```python
from build123d import *

# Parameters (mm, degrees)
EXTRU_MINCE1_DEPTH      = 25
CONG_1_R                = 1
CONG_2_R                = 1
CONG_3_R                = 2
CONG_4_R                = 2
ESQUISSE2_R             = 1.75
ENL_V_MAT_EXTRU_1_DEPTH = 2
ESQUISSE3_R             = 2.25
ENL_V_MAT_EXTRU_2_DEPTH = 2
CONG_12_R               = 2
CONG_13_R               = 2
CONG_15_R               = 2
CONG_16_R               = 2


with BuildPart() as part:
    # Esquisse1 → Extru.-Mince1 (new body)
    with BuildSketch(Plane.XY):
        Polygon((0, 45), (0, 0), (40, 0), (40, 20), (42, 20), (42, -2), (-2, -2), (-2, 45), align=None)
    extrude(amount=EXTRU_MINCE1_DEPTH)

    # Congé1
    cong_1_edges = [part.edges().sort_by_distance(p)[0] for p in [
        (0, 0, 12.5),
    ]]
    fillet(cong_1_edges, radius=CONG_1_R)

    # Congé2
    cong_2_edges = [part.edges().sort_by_distance(p)[0] for p in [
        (40, 0, 12.5),
    ]]
    fillet(cong_2_edges, radius=CONG_2_R)

    # Congé3
    cong_3_edges = [part.edges().sort_by_distance(p)[0] for p in [
        (42, -2, 12.5),
    ]]
    fillet(cong_3_edges, radius=CONG_3_R)

    # Congé4
    cong_4_edges = [part.edges().sort_by_distance(p)[0] for p in [
        (-2, -2, 12.5),
    ]]
    fillet(cong_4_edges, radius=CONG_4_R)

    # Esquisse2 → Enlèv. mat.-Extru.1 (cut)
    with BuildSketch(Plane.ZY.offset(2)):
        with Locations((12.5, 36)):
            Circle(ESQUISSE2_R)
        with Locations((12.5, 24)):
            Circle(ESQUISSE2_R)
    extrude(amount=-ENL_V_MAT_EXTRU_1_DEPTH, mode=Mode.SUBTRACT)

    # Esquisse3 → Enlèv. mat.-Extru.2 (cut)
    with BuildSketch(Plane(origin=(42, 0, 0), x_dir=(0, 0, -1), z_dir=(1, 0, 0))):
        with Locations((-12.5, 10)):
            Circle(ESQUISSE3_R)
    extrude(amount=-ENL_V_MAT_EXTRU_2_DEPTH, mode=Mode.SUBTRACT)

    # Congé12
    cong_12_edges = [part.edges().sort_by_distance(p)[0] for p in [
        (41, 20, 0),
    ]]
    fillet(cong_12_edges, radius=CONG_12_R)

    # Congé13
    cong_13_edges = [part.edges().sort_by_distance(p)[0] for p in [
        (41, 20, 25),
    ]]
    fillet(cong_13_edges, radius=CONG_13_R)

    # Congé15
    cong_15_edges = [part.edges().sort_by_distance(p)[0] for p in [
        (-1, 45, 0),
    ]]
    fillet(cong_15_edges, radius=CONG_15_R)

    # Congé16
    cong_16_edges = [part.edges().sort_by_distance(p)[0] for p in [
        (-1, 45, 25),
    ]]
    fillet(cong_16_edges, radius=CONG_16_R)


solid = part.part
```
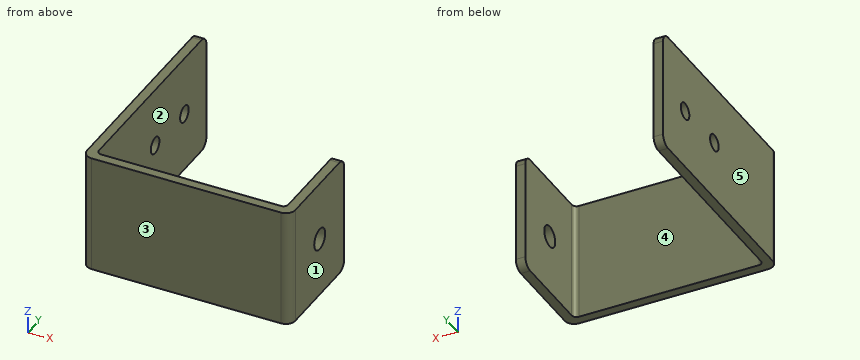
Verification items for the finished model (mm, model axes). Face numbers are marked on the shaded views. A direction names the side the tool comes from. Coordinates: 2 decimals unless noted, no trailing zeros. Loops run counter-clockwise (first coordinate to the right, second up) from the corner with the lowest first, then second, coordinate; pieces in that order, holes last. Notation, with made-up numbers: (24, -2.75) - (45, -2.75) arc R17 cw to (45, 10.25) - close; hole circle Ø6 at (-17.75, -5.5). An arc over 180 degrees is marked (long way). Put each result on its own line as item: value.
Item 1: Scan lines: line 1 along X through (y, z) = (16, 20.25); line 2 along Y through (x, z) = (-0.6, 12.5); line 3 along Y through (x, z) = (-0.8, 12.5). Record each from-to range of solid material in increasing order.
Conclusion:
line 1: x = -2 to 0, 40 to 42
line 2: y = -1.91 to 22.25, 25.75 to 34.25, 37.75 to 45
line 3: y = -1.83 to 22.25, 25.75 to 34.25, 37.75 to 45
Item 2: Draft check along X on the marked faces 3, 4 and 5. Enter one of: pulls with the +X half, pulls with the -X half, needs draft (parallel to the pull), parting line crosses it, or undercut.
Conclusion:
face 3: needs draft
face 4: undercut
face 5: pulls with the -X half
Item 3: Section check D-D (z = 22.25). Enter the section's corners in (x, y), then the cut area to 3 significant figures.
Conclusion:
outline: (-2, 0) arc R2 ccw to (0, -2) - (40, -2) arc R2 ccw to (42, 0) - (42, 20) - (40, 20) - (40, 1) arc R1 cw to (39, 0) - (1, 0) arc R1 cw to (0, 1) - (0, 45) - (-2, 45) - close
area: 217 mm2
Item 4: Set-up check for the marked faces 1 and 2: record each of +Z, -Z, +X, -X, +Y, -Y from which the full face is reachable in a straight line by a thin tool's end or side.
Conclusion:
face 1: +Z, -Z, +X, +Y, -Y
face 2: +Z, -Z, +Y
Item 5: Section check B-B (z = 12.5). Enter the section's corners in (x, y), then the cut area to 3 significant figures.
Conclusion:
outline: (-2, 0) arc R2 ccw to (0, -2) - (40, -2) arc R2 ccw to (42, 0) - (42, 7.75) - (40, 7.75) - (40, 1) arc R1 cw to (39, 0) - (1, 0) arc R1 cw to (0, 1) - (0, 22.25) - (-2, 22.25) - close; (-2, 25.75) - (0, 25.75) - (0, 34.25) - (-2, 34.25) - close; (-2, 37.75) - (0, 37.75) - (0, 45) - (-2, 45) - close; (40, 12.25) - (42, 12.25) - (42, 20) - (40, 20) - close
area: 194 mm2
Item 6: Gauge pin test, flat ends, axial feed: pin 1 Ø1 at (x, z) = (30.5, 13.5) entering from +Y; pin 2 Ø0.6 at (x, z) = (40.5, 11) entering from +Y; pin 3 Ø4 at (y, z) = (36, 12.5) entering from +X. Record the tip position at first contact, or that the pin passes through.
Conclusion:
pin 1: stops at y = 0
pin 2: stops at y = 20
pin 3: stops at x = 0
Item 7: Section check A-A (y = 24). Enter the section's corners in (x, z), then the cut area to 3 significant figures.
Conclusion:
outline: (-2, 0) - (0, 0) - (0, 10.75) - (-2, 10.75) - close; (-2, 14.25) - (0, 14.25) - (0, 25) - (-2, 25) - close
area: 43.0 mm2
Item 8: Section check C-C (y = 10). Enter the section's corners in (x, z).
Conclusion:
outline: (-2, 0) - (0, 0) - (0, 25) - (-2, 25) - close; (40, 0) - (42, 0) - (42, 10.25) - (40, 10.25) - close; (40, 14.75) - (42, 14.75) - (42, 25) - (40, 25) - close
